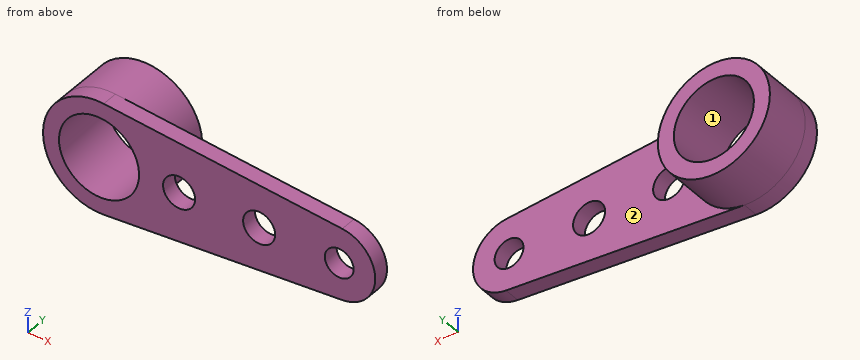
from build123d import *

# Parameters (mm, degrees)
BOSS_EXTRUDE1_DEPTH = 1
SKETCH2_R           = 3.5
BOSS_EXTRUDE2_DEPTH = 3
SKETCH3_R           = 2.5
CUT_EXTRUDE1_DEPTH  = 19.050277006
SKETCH4_R           = 0.9
CUT_EXTRUDE2_DEPTH  = 19.050277006
CUT_EXTRUDE3_DEPTH  = 19.050277006


with BuildPart() as part:
    # Sketch1 → Boss-Extrude1 (new body)
    with BuildSketch(Plane(origin=(0, 0, 0), x_dir=(1, 0, 0), z_dir=(0, 1, 0))):
        with BuildLine():
            Line((15.1875, 2.242173889), (0.291666667, 3.48782605))
            ThreePointArc((0.291666667, 3.48782605), (-3.5, 0), (0.291666667, -3.48782605))
            Line((0.291666667, -3.48782605), (15.1875, -2.242173889))
            ThreePointArc((15.1875, -2.242173889), (17.25, 0), (15.1875, 2.242173889))
        make_face()
    extrude(amount=BOSS_EXTRUDE1_DEPTH)

    # Sketch2 → Boss-Extrude2 (add)
    with BuildSketch(Plane(origin=(0, 1, 0), x_dir=(1, 0, 0), z_dir=(0, 1, 0))):
        with Locations(Location((0, 0, 0), (0, 0, 85.219808153))):
            Circle(SKETCH2_R)
    extrude(amount=BOSS_EXTRUDE2_DEPTH)

    # Sketch3 → Cut-Extrude1 (cut, through all)
    with BuildSketch(Plane(origin=(0, 4, 0), x_dir=(1, 0, 0), z_dir=(0, 1, 0))):
        with Locations(Location((0, 0, 0), (0, 0, 270))):
            Circle(SKETCH3_R)
    extrude(amount=-CUT_EXTRUDE1_DEPTH, mode=Mode.SUBTRACT)

    # Sketch4 → Cut-Extrude2 (cut, through all)
    with BuildSketch(Plane.XZ):
        with Locations(Location((15, 0, 0), (0, 0, 270))):
            Circle(SKETCH4_R)
    extrude(amount=-CUT_EXTRUDE2_DEPTH, mode=Mode.SUBTRACT)

    # Sketch5 → Cut-Extrude3 (cut, through all)
    with BuildSketch(Plane.XZ):
        with BuildLine():
            ThreePointArc((6, 0), (5, 1), (4, 0))
            Line((4, 0), (6, 0))
        make_face()
        with BuildLine():
            Line((6, 0), (4, 0))
            ThreePointArc((4, 0), (5, -1), (6, 0))
        make_face()
        with BuildLine():
            ThreePointArc((11, 0), (10, 1), (9, 0))
            Line((9, 0), (11, 0))
        make_face()
        with BuildLine():
            Line((11, 0), (9, 0))
            ThreePointArc((9, 0), (10, -1), (11, 0))
        make_face()
    extrude(amount=-CUT_EXTRUDE3_DEPTH, mode=Mode.SUBTRACT)


solid = part.part
For this review, take the finished solid that the model builds, in its own axes (mm). Face numbers are marked on the shaded views. Round coordinates to 2 decimals unless told otherwise and drop trailing zeros. Order: outer loops, then holes, each group sorted by start corner. A loop starts at its lowest first (then second) coordinate and runs counter-clockwise, first axis right, second up. Notation, with made-up numbers: (10.5, -4) -> (16.5, -4) arc R17 ccw to (16.5, 5) -> close; hole circle Ø10 at (43.25, -33.5). An arc over 180 degrees is marked (long way). Write item = value, one per line. Start each with the question number.
1) Take a section at A-A on z = 0. State the section outline as (x, y) points, plus the area to 4 significant figures.
2) Insertion check: pin 1 (2.5 mm diameter, centred on x = 5, z = 0, fed in from +Y); pin 2 (4 mm diameter, centred on x = 1, z = 1, fed in from -Y); pin 3 (2 mm diameter, centred on x = 13, y = 1.5, fed in from +Z); pin 4 (1 mm diameter, centred on y = 3, z = 0, fed in from +X). Each pin has a flat end and moves straight along its axis. Give the tip position at first contact, or say it passes through.
3) Take a section at D-D on z = 3.25. State the section outline as (x, y) points, plus the area to 3 significant figures.
4) Take a section at B-B on x = 0. State the section outline as (y, z) points, plus the area to 3 significant figures.
5) To check wall thickness, follow line 1 (X direction, y = 0.7, z = 0); line 2 (Y direction, x = 3.75, z = -1.5); line 3 (Z direction, x = 10, y = 0.5). State the ranges of each line that lie inside material, in increasing order. Write a range as from..to.
6) The part is to be moulded in two halves that separate along X. For the marked faces 1 and 2, say which applies: +X half, -X half, draft (parallel to the pull), parting line (faces both ways), or undercut.
7) Take a section at C-C on y = 0.3. State the section outline as (x, z) points.
Verdict:
q1.outline = (-3.5, 0) -> (-2.5, 0) -> (-2.5, 4) -> (-3.5, 4) -> close; (2.5, 0) -> (4, 0) -> (4, 1) -> (3.5, 1) -> (3.5, 4) -> (2.5, 4) -> close; (6, 0) -> (9, 0) -> (9, 1) -> (6, 1) -> close; (11, 0) -> (14.1, 0) -> (14.1, 1) -> (11, 1) -> close; (15.9, 0) -> (17.25, 0) -> (17.25, 1) -> (15.9, 1) -> close
q1.area = 15.95 mm2
q2.pin_1 = 1
q2.pin_2 = 0
q2.pin_3 = 2.5
q2.pin_4 = 3.5
q3.outline = (-1.3, 0) -> (3.14, 0) -> (3.14, 1) -> (1.3, 1) -> (1.3, 4) -> (-1.3, 4) -> close
q3.area = 12.2 mm2
q4.outline = (0, -3.5) -> (4, -3.5) -> (4, -2.5) -> (0, -2.5) -> close; (0, 2.5) -> (4, 2.5) -> (4, 3.5) -> (0, 3.5) -> close
q4.area = 8.00 mm2
q5.line_1 = -3.5..-2.5, 2.5..4, 6..9, 11..14.1, 15.9..17.25
q5.line_2 = 0..1
q5.line_3 = -2.68..-1, 1..2.68
q6.face_1 = undercut
q6.face_2 = draft
q7.outline = (0.29, -3.49) -> (15.19, -2.24) arc R2.25 ccw to (15.19, 2.24) -> (0.29, 3.49) arc R3.5 ccw (long way) to start; hole circle Ø5 at (0, 0); hole circle Ø2 at (5, 0); hole circle Ø2 at (10, 0); hole circle Ø1.8 at (15, 0)
